Input: part model. Units: mm. Frame: model coordinates. Round coordinates to 2 decimals unless told otherwise and drop trailing zeros. Write each loop counter-clockwise with the first axis right and the second up, starting at its lowest first coordinate (ties: lowest second). Pieces come first, ordered by that corner, then holes. Notation, with made-up numbers: M -28,1.5 L 24,1.5 A15 ccw 24,6.5 Z; hole C -20.75,-40 d6. An arc over 180 degrees is marked long. Answer as CSV lines item,"result". Start each with the question number.
```python
from build123d import *

# Parameters (mm, degrees)
ENL_V_MAT_EXTRU_3_DEPTH      = 64.710281815
ENL_V_MAT_EXTRU_3_DEPTH_BACK = 64.710281815
ENL_V_MAT_EXTRU_8_DEPTH      = 64.921827328
ENL_V_MAT_EXTRU_8_DEPTH_BACK = 64.921827328


with BuildPart() as part:
    # Esquisse2 → Révolution1 (revolve)
    with BuildSketch(Plane(origin=(0, 0, 0), x_dir=(0, 0, -1), z_dir=(1, 0, 0)), mode=Mode.PRIVATE) as r_volution1_sk:
        with BuildLine():
            Line((3, 0), (-3, 0))
            Line((-3, 0), (-3, 43.5))
            ThreePointArc((-3, 43.5), (-2.560660172, 44.560660172), (-1.5, 45))
            Line((-1.5, 45), (-1.3, 45))
            ThreePointArc((-1.3, 45), (0, 43.7), (1.3, 45))
            Line((1.3, 45), (1.5, 45))
            ThreePointArc((1.5, 45), (2.560660172, 44.560660172), (3, 43.5))
            Line((3, 43.5), (3, 0))
        make_face()
    revolve(r_volution1_sk.sketch.rotate(Axis((0, 0, 77.254476924), (0, 0, -1)), 90), axis=Axis((0, 0, 77.254476924), (0, 0, -1)))

    # Esquisse3 → Enlèv. mat.-Extru.3 (cut, two sides: drawn at the far end of the back side and taken through both)
    with BuildSketch(Plane.XY.offset(-ENL_V_MAT_EXTRU_3_DEPTH_BACK)):
        with BuildLine():
            Line((-1.209338662, 2.8), (1.209338662, 2.8))
            ThreePointArc((1.209338662, 2.8), (0, -3.05), (-1.209338662, 2.8))
        make_face()
    extrude(amount=ENL_V_MAT_EXTRU_3_DEPTH + ENL_V_MAT_EXTRU_3_DEPTH_BACK, mode=Mode.SUBTRACT)

    # Esquisse5 → Enlèv. mat.-Extru.8 (cut, two sides: drawn at the far end of the back side and taken through both)
    with BuildSketch(Plane.XY.offset(3).offset(-ENL_V_MAT_EXTRU_8_DEPTH_BACK)):
        with BuildLine():
            ThreePointArc((-10.434150973, 7.754256475), (-11.222640125, 6.561428855), (-11.875358384, 5.289221422))
            ThreePointArc((-11.875358384, 5.289221422), (-14.082795768, 2.915548976), (-17.282106883, 2.394483639))
            Line((-17.282106883, 2.394483639), (-32.821462414, 5.040473711))
            ThreePointArc((-32.821462414, 5.040473711), (-36.244832016, 7.356172767), (-36.755616081, 11.457516594))
            ThreePointArc((-36.755616081, 11.457516594), (-32.932247903, 19.942844532), (-27.184402598, 27.262763165))
            ThreePointArc((-27.184402598, 27.262763165), (-23.229227503, 28.704072082), (-19.575116576, 26.61403506))
            Line((-19.575116576, 26.61403506), (-10.368441836, 13.6285533))
            ThreePointArc((-10.368441836, 13.6285533), (-9.447598742, 10.680736947), (-10.434150973, 7.754256475))
        make_face()
        with BuildLine():
            ThreePointArc((-11.932458581, -5.159111572), (-11.293684136, -6.438377019), (-10.51827931, -7.639751328))
            ThreePointArc((-10.51827931, -7.639751328), (-9.566337363, -10.738284404), (-10.714737101, -13.769501772))
            Line((-10.714737101, -13.769501772), (-20.775909487, -25.903983384))
            ThreePointArc((-20.775909487, -25.903983384), (-24.493048499, -27.710858898), (-28.300308475, -26.102538961))
            ThreePointArc((-28.300308475, -26.102538961), (-33.73713394, -18.548741022), (-37.202446777, -9.911001654))
            ThreePointArc((-37.202446777, -9.911001654), (-36.473069367, -5.765065087), (-32.835988747, -3.645530707))
            Line((-32.835988747, -3.645530707), (-16.986894292, -2.165057378))
            ThreePointArc((-16.986894292, -2.165057378), (-13.973588898, -2.841492042), (-11.932458581, -5.159111572))
        make_face()
        with BuildLine():
            ThreePointArc((-1.498307609, -12.913368047), (-0.071044011, -12.999805873), (1.357079074, -12.928972751))
            ThreePointArc((1.357079074, -12.928972751), (4.516458405, -13.65383338), (6.567369781, -16.163985411))
            Line((6.567369781, -16.163985411), (12.045552926, -30.944457095))
            ThreePointArc((12.045552926, -30.944457095), (11.751783517, -35.067031665), (8.455307606, -37.560055555))
            ThreePointArc((8.455307606, -37.560055555), (-0.804886037, -38.491585554), (-10.018044179, -37.173764819))
            ThreePointArc((-10.018044179, -37.173764819), (-13.243841863, -34.469137169), (-13.260872171, -30.259565767))
            Line((-13.260872171, -30.259565767), (-6.618452456, -15.793610677))
            ThreePointArc((-6.618452456, -15.793610677), (-4.525990156, -13.522228989), (-1.498307609, -12.913368047))
        make_face()
        with BuildLine():
            ThreePointArc((10.434150973, -7.754256475), (11.222640125, -6.561428855), (11.875358384, -5.289221422))
            ThreePointArc((11.875358384, -5.289221422), (14.082795768, -2.915548976), (17.282106883, -2.394483639))
            Line((17.282106883, -2.394483639), (32.821462414, -5.040473711))
            ThreePointArc((32.821462414, -5.040473711), (36.244832016, -7.356172767), (36.755616081, -11.457516594))
            ThreePointArc((36.755616081, -11.457516594), (32.932247903, -19.942844532), (27.184402598, -27.262763165))
            ThreePointArc((27.184402598, -27.262763165), (23.229227503, -28.704072082), (19.575116576, -26.61403506))
            Line((19.575116576, -26.61403506), (10.368441836, -13.6285533))
            ThreePointArc((10.368441836, -13.6285533), (9.447598742, -10.680736947), (10.434150973, -7.754256475))
        make_face()
        with BuildLine():
            ThreePointArc((11.932458581, 5.159111572), (11.293684136, 6.438377019), (10.51827931, 7.639751328))
            ThreePointArc((10.51827931, 7.639751328), (9.566337363, 10.738284404), (10.714737101, 13.769501772))
            Line((10.714737101, 13.769501772), (20.775909487, 25.903983384))
            ThreePointArc((20.775909487, 25.903983384), (24.493048499, 27.710858898), (28.300308475, 26.102538961))
            ThreePointArc((28.300308475, 26.102538961), (33.73713394, 18.548741022), (37.202446777, 9.911001654))
            ThreePointArc((37.202446777, 9.911001654), (36.473069367, 5.765065087), (32.835988747, 3.645530707))
            Line((32.835988747, 3.645530707), (16.986894292, 2.165057378))
            ThreePointArc((16.986894292, 2.165057378), (13.973588898, 2.841492042), (11.932458581, 5.159111572))
        make_face()
        with BuildLine():
            Line((-12.045552926, 30.944457095), (-6.567369781, 16.163985411))
            ThreePointArc((-6.567369781, 16.163985411), (-4.516458405, 13.65383338), (-1.357079074, 12.928972751))
            ThreePointArc((-1.357079074, 12.928972751), (0.071044011, 12.999805873), (1.498307609, 12.913368047))
            ThreePointArc((1.498307609, 12.913368047), (4.525990156, 13.522228989), (6.618452456, 15.793610677))
            Line((6.618452456, 15.793610677), (13.260872171, 30.259565767))
            ThreePointArc((13.260872171, 30.259565767), (13.243841863, 34.469137169), (10.018044179, 37.173764819))
            ThreePointArc((10.018044179, 37.173764819), (0.804886037, 38.491585554), (-8.455307606, 37.560055555))
            ThreePointArc((-8.455307606, 37.560055555), (-11.751783517, 35.067031665), (-12.045552926, 30.944457095))
        make_face()
    extrude(amount=ENL_V_MAT_EXTRU_8_DEPTH + ENL_V_MAT_EXTRU_8_DEPTH_BACK, mode=Mode.SUBTRACT)


solid = part.part
```
Item 1: Cut plane A-A, the plane x = 0. Return loops of the section in (y, z), plus the area to 3 significant figures.
Item 2: Pin query (flat end, axial travel): pin 1 Ø2.5 at (x, z) = (-0.5, -0.5) entering from -Y; pin 2 Ø3 at (y, z) = (-27.5, 0.5) entering from -X; pin 3 Ø3 at (y, z) = (28.5, -2.5) entering from -X. Return the tip coordinate at first contact, or that it passes through.
Item 3: Line query: line 1 (Y direction, x = 0, z = 1.7); line 2 (X direction, y = 21, z = -0.5); line 3 (Y direction, x = 0, z = 0.95). Output: solid intervals per line, ascending. Write a range as [from, to].
Item 4: Cut plane C-C, the plane z = 0.25. Give the number of separate pieces and of enclosed holes in the cut face, plus the area to 3 significant figures.
Item 5: Cut plane B-B, the plane y = 0. Return loops of the section in (x, z), plus the area to 3 significant figures.
Item 6: Draft query along X for faces 1 (the face through (0.94, 38.49, -0.04)), 2 (the face through (-0.674, -38.494, -0.042)). Return one class per face: +X half, -X half, draft (parallel to the pull), parting line (faces both ways), or undercut.
Results list:
1,outline,"M -45,-1.5 A1.5 ccw -43.5,-3 L -38.5,-3 L -38.5,3 L -43.5,3 A1.5 ccw -45,1.5 L -45,1.3 A1.3 cw -45,-1.3 Z; M -13,-3 L -3.05,-3 L -3.05,3 L -13,3 Z; M 2.8,-3 L 13,-3 L 13,3 L 2.8,3 Z; M 38.5,-3 L 43.5,-3 A1.5 ccw 45,-1.5 L 45,-1.3 A1.3 cw 45,1.3 L 45,1.5 A1.5 ccw 43.5,3 L 38.5,3 Z"
1,area,"192 mm²"
2,pin 1,"y = -45"
2,pin 2,"x = -36.56"
2,pin 3,"x = -35.84"
3,line 1,"[-44.99, -38.5], [-13, -3.05], [2.8, 13], [38.5, 44.99]"
3,line 2,"[-38.44, -32.27], [-15.59, -8.36], [9.01, 16.71], [32.27, 38.44]"
3,line 3,"[-44.11, -38.5], [-13, -3.05], [2.8, 13], [38.5, 44.11]"
4,separate pieces,"1"
4,enclosed holes,"7"
4,area,"3,010 mm²"
5,outline,"M -45,-1.5 A1.5 ccw -43.5,-3 L -3.05,-3 L -3.05,3 L -43.5,3 A1.5 ccw -45,1.5 L -45,1.3 A1.3 cw -45,-1.3 Z; M 3.05,-3 L 43.5,-3 A1.5 ccw 45,-1.5 L 45,-1.3 A1.3 cw 45,1.3 L 45,1.5 A1.5 ccw 43.5,3 L 3.05,3 Z"
5,area,"496 mm²"
6,face 1,"undercut"
6,face 2,"undercut"
